from build123d import *

# Parameters (mm, degrees)
F0_W     = 20
F0_H     = 25.4
F1_DEPTH = 5
F2_T     = -1.524
F3_R     = 1.25
F3_R_2   = 1.2446
F4_DEPTH = 25.4


with BuildPart() as f1:
    # F0 (on Front) → F1 (new body)
    with BuildSketch(Plane.XZ):
        Rectangle(F0_W, F0_H)
    extrude(amount=F1_DEPTH)

    # F2
    f2_openings = [f1.faces().sort_by_distance(p)[0] for p in [
        (0, 0, 0),
    ]]
    offset(amount=F2_T, openings=f2_openings)

    # F3 (on face) → F4 (cut)
    with BuildSketch(Plane.YZ.offset(10)):
        with Locations((-1.952, 8.89)):
            Circle(F3_R)
        with Locations((-1.952, -8.89)):
            Circle(F3_R_2)
    extrude(amount=-F4_DEPTH, mode=Mode.SUBTRACT)


solid = f1.part
The model under review builds one solid part; all positions refer to its coordinate system, in mm. A direction names the side the tool comes from. Give positions to 0.01 mm unless a question says otherwise; leave off trailing zeros. Write each loop counter-clockwise with the first axis right and the second up, starting at its lowest first coordinate (ties: lowest second). Pieces come first, ordered by that corner, then holes.
1. Add section B-B, the plane x = -6. Write out the cut boundary in (y, z), plus the area to 3 significant figures.
2. Wall thickness on L1, parallel to X at y = -1.35, z = -11; L2, parallel to Z at x = 3, y = -2.25; L3, parallel to Y at x = 3, z = 4.75: over which ranges is each line inside the solid? List them lowest first.
3. Add section C-C, the plane z = 5.75. Write out the cut boundary in (x, y).
4. Add section D-D, the plane z = 8.89. Write out the cut boundary in (x, y), plus the area to 3 significant figures.
5. For P1, Ø5, axis at x = 1.5, z = -3, coming from the +Y side, flat-tipped, find the tip position at first contact; note if it passes through.
6. Add section A-A, the plane z = -8.89. Write out the cut boundary in (x, y), plus the area to 3 significant figures.
7. Tool access review of faces 5 (the flat face through (0, -2, -11.176)), 6 (the flat face through (0, -2, 12.7)): name each direction out of +Z, -Z, +X, -X, +Y, -Y from which nothing blocks a thin tool from reaching the whole face with its end or side.
8. Draft analysis for pull direction X (two halves, no side actions). For faces 1 (the flat face through (10, -2, 0)), 2 (the flat face through (8.476, -2, 0)), 3 (the cylindrical face through (9.249, -1.28, 9.944)), 4 (the flat face through (0, -3.476, 0)), state which applies: +X half, -X half, draft (parallel to the pull), parting line (faces both ways), or undercut.
Worked answers:
1. outline: (-5, -12.7) - (0, -12.7) - (0, -11.18) - (-3.48, -11.18) - (-3.48, 11.18) - (0, 11.18) - (0, 12.7) - (-5, 12.7) - close
1. area: 49.3 mm2
2. L1: x = -10 to -8.48, 8.48 to 10
2. L2: z = -12.7 to -11.18, 11.18 to 12.7
2. L3: y = -5 to -3.48
3. outline: (-10, -5) - (10, -5) - (10, 0) - (8.48, 0) - (8.48, -3.48) - (-8.48, -3.48) - (-8.48, 0) - (-10, 0) - close
4. outline: (-10, -5) - (10, -5) - (10, -3.2) - (8.48, -3.2) - (8.48, -3.48) - (-8.48, -3.48) - (-8.48, -3.2) - (-10, -3.2) - close; (-10, -0.7) - (-8.48, -0.7) - (-8.48, 0) - (-10, 0) - close; (8.48, -0.7) - (10, -0.7) - (10, 0) - (8.48, 0) - close
4. area: 33.5 mm2
5. P1: stops at y = -3.48
6. outline: (-10, -5) - (10, -5) - (10, -3.2) - (8.48, -3.2) - (8.48, -3.48) - (-8.48, -3.48) - (-8.48, -3.2) - (-10, -3.2) - close; (-10, -0.71) - (-8.48, -0.71) - (-8.48, 0) - (-10, 0) - close; (8.48, -0.71) - (10, -0.71) - (10, 0) - (8.48, 0) - close
6. area: 33.5 mm2
7. face 5: +Y
7. face 6: +Z, +X, -X, +Y, -Y
8. face 1: +X half
8. face 2: undercut
8. face 3: draft
8. face 4: undercut
